CAD build for the part. Positions are in the model's coordinates, mm. Face numbers are marked on the shaded views. A direction names the side the tool comes from. Round coordinates to 2 decimals unless told otherwise and drop trailing zeros. Loops run counter-clockwise (first coordinate to the right, second up) from the corner with the lowest first, then second, coordinate; pieces in that order, holes last. Notation, with made-up numbers: (2.25, 88.25) - (43.25, 88.25) arc R20 cw to (43.25, 97.25) - close; hole circle Ø3 at (31, 89). An arc over 180 degrees is marked (long way). Use one line per item in the form item = value.
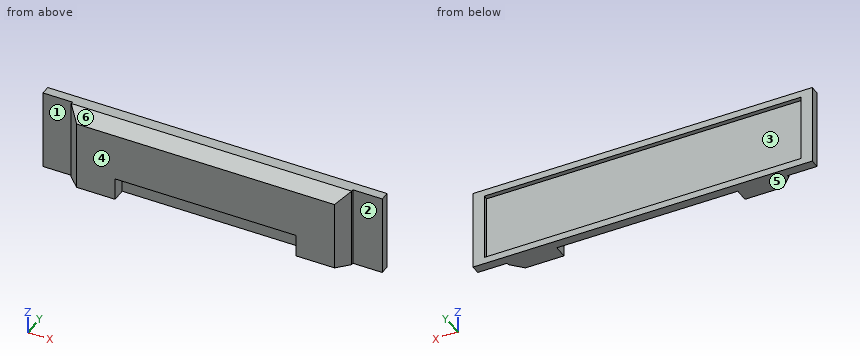
from build123d import *

# Parameters (mm, degrees)
F0_W     = 750
F0_H     = 180
F1_DEPTH = 20
F2_W     = 620
F2_H     = 180
F3_DEPTH = 30
F4_SIZE  = 25
F5_W     = 400
F5_H     = 50
F6_DEPTH = 30
F7_W     = 700
F7_H     = 150
F8_DEPTH = 10


with BuildPart() as f1:
    # F0 (on Front) → F1 (new body)
    with BuildSketch(Plane.XZ):
        Rectangle(F0_W, F0_H)
    extrude(amount=F1_DEPTH)

    # F2 (on face) → F3 (join)
    with BuildSketch(Plane.XZ.offset(20)):
        Rectangle(F2_W, F2_H)
    extrude(amount=F3_DEPTH)

    # F4
    f4_edges = [f1.edges().sort_by_distance(p)[0] for p in [
        (0, -50, 90),
        (-310, -50, 0),
        (310, -50, 0),
    ]]
    chamfer(f4_edges, length=F4_SIZE)

    # F5 (on face) → F6 (cut)
    with BuildSketch(Plane.XZ.offset(50)):
        with Locations((0, -65)):
            Rectangle(F5_W, F5_H)
    extrude(amount=-F6_DEPTH, mode=Mode.SUBTRACT)

    # F7 (on face) → F8 (cut)
    with BuildSketch(Plane(origin=(0, 0, 0), x_dir=(-1, 0, 0), z_dir=(0, 1, 0))):
        Rectangle(F7_W, F7_H)
    extrude(amount=-F8_DEPTH, mode=Mode.SUBTRACT)


solid = f1.part
1) Flat gauge pins, fed straight in: pin 1 (12 mm diameter, centred on x = -91, y = -25.5, fed in from -Z); pin 2 (24 mm diameter, centred on x = 35.5, y = -40.5, fed in from -Z); pin 3 (12 mm diameter, centred on y = -39.5, z = 2, fed in from -X); pin 4 (1.5 mm diameter, centred on y = -22, z = -39, fed in from -X). Where does each tip first touch, or does it go through?
Report:
pin_1 = -90
pin_2 = -40
pin_3 = -301.5
pin_4 = -310
2) Slice it at C-C (z = 42.5). Write the cut outline in (x, y), plus the area to 3 significant figures.
Report:
outline = (-375, -20) - (-310, -20) - (-310, -25) - (-285, -50) - (285, -50) - (310, -25) - (310, -20) - (375, -20) - (375, 0) - (350, 0) - (350, -10) - (-350, -10) - (-350, 0) - (-375, 0) - close
area = 26,000 mm^2
3) Two-plate mould, pull along Z, no slides. Class the marked faces 3, 4, 5 and 6: +Z half, -Z half, draft (parallel to the pull), parting line (faces both ways), or undercut.
Report:
face_3 = undercut
face_4 = draft
face_5 = -Z half
face_6 = +Z half
4) Tool access for the marked faces 1 and 2: list every direction of +Z, -Z, +X, -X, +Y, -Y with a clear straight run to the whole face (end or side of a thin tool).
Report:
face_1 = +Z, -Z, -X, -Y
face_2 = +Z, -Z, +X, -Y
5) Slice it at D-D (x = 178.5). Write the cut outline in (y, z).
Report:
outline = (-50, -40) - (-20, -40) - (-20, -90) - (0, -90) - (0, -75) - (-10, -75) - (-10, 75) - (0, 75) - (0, 90) - (-25, 90) - (-50, 65) - close
6) Slice it at B-B (x = 277.5). Write the cut outline in (y, z), plus the area to 3 significant figures.
Report:
outline = (-50, -90) - (0, -90) - (0, -75) - (-10, -75) - (-10, 75) - (0, 75) - (0, 90) - (-25, 90) - (-50, 65) - close
area = 7,190 mm^2
7) Slice it at A-A (y = -41.5). Write the cut outline in (x, z), plus the area to 3 significant figures.
Report:
outline = (-293.5, -90) - (-200, -90) - (-200, -40) - (200, -40) - (200, -90) - (293.5, -90) - (293.5, 73.5) - (-293.5, 73.5) - close
area = 76,000 mm^2
8) Drill centre lines: probe 1 along Z at (x, y) = (222, -6.5); probe 2 along Y at (x, z) = (319, -43.5); probe 3 along Z at (x, y) = (-70, -22). Where is each one in solid material? Low to high.
Report:
probe_1 = -90 to -75, 75 to 90
probe_2 = -20 to -10
probe_3 = -40 to 90
